from build123d import *

# Parameters (mm, degrees)
SKETCH_1_R          = 1.55
EXTRUDE_511_DEPTH   = 2.5
EXTRUDE_START       = 2.5
EXTRUDE_978_DEPTH   = 7.5
SKETCH_3_W          = 4.5
SKETCH_3_H          = 12.978713764
EXTRUDE_1_DEPTH     = 9.75
CHAMFER_1_SIZE      = 1
FILLET_5_R          = 0.75
CUT_EXTRUDE_1_DEPTH = 2
SKETCH_7_R          = 1.55
CUT_EXTRUDE_2_DEPTH = 4.5
FILLET_6_R          = 0.25


with BuildPart() as part:
    # 草图1 → Extrude 511 (new body)
    with BuildSketch(Plane(origin=(0, 0, 0), x_dir=(1, 0, 0), z_dir=(0, 1, 0))):
        with BuildLine():
            Line((-10.1243866, 13.845154317), (6.15423406, 2.01804411))
            ThreePointArc((6.15423406, 2.01804411), (7.315700706, -5.315167685), (-0.017511089, -6.476634331))
            Line((-0.017511089, -6.476634331), (-10.1243866, 0.866440553))
            Line((-10.1243866, 0.866440553), (-10.1243866, 13.845154317))
        make_face()
        with Locations(Location((0, 0, 0), (0, 0, 270))):
            Circle(SKETCH_1_R, mode=Mode.SUBTRACT)
    extrude(amount=EXTRUDE_511_DEPTH)

    # 草图2 → Extrude 978 (add)
    with BuildSketch(Plane(origin=(0, 0, 0), x_dir=(1, 0, 0), z_dir=(0, 1, 0)).offset(EXTRUDE_START)):
        Polygon((-10.1243866, 0.866440553), (-0.017511089, -6.476634331), (-1.193081594, -8.09466832), (-11.299957105, -0.751593436), align=None)
        Polygon((7.329804565, 3.636078099), (-0.809505765, 9.549633202), (-1.98507627, 7.931599213), (6.15423406, 2.01804411), align=None)
    extrude(amount=-EXTRUDE_978_DEPTH)

    # 草图3 → 限位-1 (add)
    with BuildSketch(Plane(origin=(0, 0, 0), x_dir=(1, 0, 0), z_dir=(0, 1, 0))):
        with Locations((-12.3743866, 7.355797435)):
            Rectangle(SKETCH_3_W, SKETCH_3_H)
    extrude(amount=EXTRUDE_1_DEPTH)

    # 倒角1
    chamfer_1_edges = [part.edges().sort_by_distance(p)[0] for p in [
        (0, 0, -1.55),
        (0, 2.5, -1.55),
    ]]
    chamfer(chamfer_1_edges, length=CHAMFER_1_SIZE)

    # 圆角5
    fillet_5_edges = [part.edges().sort_by_distance(p)[0] for p in [
        (-1.193081594, -1.25, 8.09466832),
        (-11.299957105, -1.25, 0.751593436),
        (-1.98507627, 1.25, -7.931599213),
        (-0.809505765, -1.25, -9.549633202),
        (7.329804565, -1.25, -3.636078099),
        (-0.017511089, 1.25, 6.476634331),
        (6.15423406, 1.25, -2.01804411),
    ]]
    fillet(fillet_5_edges, radius=FILLET_5_R)

    # 草图5 → 切除-拉伸1 (cut)
    with BuildSketch(Plane(origin=(-10.1243866, 0, 0), x_dir=(0, 0, -1), z_dir=(1, 0, 0))):
        Polygon((10.560091429, 5.75), (8.957944432, 8.525), (5.753650438, 8.525), (4.151503441, 5.75), (5.753650438, 2.975), (8.957944432, 2.975), align=None)
    extrude(amount=-CUT_EXTRUDE_1_DEPTH, mode=Mode.SUBTRACT)

    # 草图7 → 切除-拉伸2 (cut)
    with BuildSketch(Plane(origin=(-10.1243866, 0, 0), x_dir=(0, 0, -1), z_dir=(1, 0, 0))):
        with Locations((7.355797435, 5.75)):
            Circle(SKETCH_7_R)
    extrude(amount=-CUT_EXTRUDE_2_DEPTH, mode=Mode.SUBTRACT)

    # 圆角6
    fillet_6_edges = [part.edges().sort_by_distance(p)[0] for p in [
        (-10.1243866, 1.25, -0.866440553),
    ]]
    fillet(fillet_6_edges, radius=FILLET_6_R)


solid = part.part
Source: CAD feature listing. Evaluate the final solid. Frame: model axes, mm. A direction names the side the tool comes from. Coordinates: 2 decimals unless noted, no trailing zeros. Loops run counter-clockwise (first coordinate to the right, second up) from the corner with the lowest first, then second, coordinate; pieces in that order, holes last. Notation, with made-up numbers: (60.5, 39) - (77.5, 39) arc R17 ccw to (77.5, 54) - close; hole circle Ø7 at (-20.75, 79.25). An arc over 180 degrees is marked (long way). One line per item, written item: value. Start each with the question number.
1. Section B-B (z = -5). Return the cut outline in (x, y), and give its area (3 significant figures).
2. Ray query, L1, parallel to X at y = 6.25, z = -4; L2, parallel to Y at x = -13, z = -1; L3, parallel to X at y = 1.35, z = 0. Return the intervals inside material, ascending.
3. Section D-D (x = -8.5). Return the cut outline in (y, z), and give its area (3 significant figures).
4. Contact query for flat-ended pins moving along their axis: P1, Ø0.6, axis at x = -11, z = -7, coming from the -Y side; P2, Ø1.3, axis at x = -12.5, y = 7, coming from the +Z side; P3, Ø1, axis at x = -1, z = -7.5, coming from the +Y side. Output: stop coordinate, or through.
5. Section A-A (y = -1.25). Return the cut outline in (x, z), and give its area (3 significant figures).
6. Set-up query: faces 4 (the flat face through (-1.613, -2.031, -8.444)), 5 (the flat face through (-11.11, 4.343, -9.748)), 6 (the flat face through (-6.18, -1.2, 4.47)). Return all of +Z, -Z, +X, -X, +Y, -Y with unobstructed straight access to the full face (end or side cutting, diameter ignored); none if empty.
7. Mould query, pull axis Y, two halves, no side actions, for faces 1 (the cylindrical face through (-1.234, -1.303, 7.786)), 2 (the flat face through (-11.11, 7.157, -4.964)), 3 (the flat face through (-12, 9.75, -7)). Classes: pulls with the +Y half, pulls with the -Y half, needs draft (parallel to the pull), parting line crosses it, or undercut.
8. Section C-C (y = 3.75). Return the cut outline in (x, z).
Verdict:
1. outline: (-14.62, 0) - (2.05, 0) - (2.05, -5) - (5.45, -5) - (5.45, 2.5) - (-10.12, 2.5) - (-10.12, 4.28) - (-12.12, 4.28) - (-12.12, 7.22) - (-10.12, 7.22) - (-10.12, 9.75) - (-14.62, 9.75) - close
1. area: 94.0 mm2
2. L1: x = -14.62 to -10.12
2. L2: y = 0 to 9.75
2. L3: x = -10.75 to -1.55, 1.55 to 7.82
3. outline: (-5, 0.31) - (0, 0.31) - (0, -12.66) - (2.5, -12.66) - (2.5, 2.79) - (-5, 2.79) - close
3. area: 51.0 mm2
4. P1: stops at y = 0
4. P2: stops at z = -0.87
4. P3: stops at y = 2.5
5. outline: (-10.86, 0.14) - (-10.12, -0.87) - (-0.02, 6.48) - (-0.75, 7.49) arc R0.75 ccw to (-1.8, 7.65) - (-10.69, 1.19) arc R0.75 ccw to start; (-1.99, -7.93) - (-1.25, -8.94) arc R0.75 ccw to (-0.2, -9.11) - (6.72, -4.08) arc R0.75 ccw to (6.89, -3.03) - (6.15, -2.02) - close
5. area: 44.6 mm2
6. face 4: -Z, -Y
6. face 5: +X
6. face 6: +Z, -X, +Y, -Y
7. face 1: needs draft
7. face 2: undercut
7. face 3: pulls with the +Y half
8. outline: (-14.62, -13.85) - (-10.12, -13.85) - (-10.12, -9.41) - (-12.12, -9.41) - (-12.12, -5.31) - (-10.12, -5.31) - (-10.12, -0.87) - (-14.62, -0.87) - close
